CAD build for the part. Positions are in the model's coordinates, mm. A direction names the side the tool comes from. Give positions to 0.01 mm unless a question says otherwise; leave off trailing zeros. Loops run counter-clockwise (first coordinate to the right, second up) from the corner with the lowest first, then second, coordinate; pieces in that order, holes last. Notation, with made-up numbers: (17.25, 71.5) -> (55.25, 71.5) arc R26 cw to (55.25, 107.5) -> close; hole circle Ø2 at (-27, 24.5). An arc over 180 degrees is marked (long way). Use one line per item in the form item = value.
```python
from build123d import *

# Parameters (mm, degrees)
SKETCH1_R           = 77.4600051
BOSS_EXTRUDE1_DEPTH = 3.175
SKETCH24_R          = 22.1615
SKETCH24_R_2        = 2.0193
CUT_EXTRUDE14_DEPTH = 110.590991442


with BuildPart() as part:
    # Sketch1 → Boss-Extrude1 (new body)
    with BuildSketch(Plane(origin=(0, 0, 0), x_dir=(1, 0, 0), z_dir=(0, 1, 0))):
        with Locations(Location((0, 0, 0), (0, 0, 270))):
            Circle(SKETCH1_R)
    extrude(amount=BOSS_EXTRUDE1_DEPTH)

    # Sketch24 → Cut-Extrude14 (cut, through all)
    with BuildSketch(Plane(origin=(0, 3.175, 0), x_dir=(1, 0, 0), z_dir=(0, 1, 0))):
        with Locations(Location((0, 0, 0), (0, 0, 270))):
            Circle(SKETCH24_R)
        with Locations(Location((-25.4, 25.4, 0), (0, 0, 270))):
            Circle(SKETCH24_R_2)
        with Locations(Location((0, 33.02, 0), (0, 0, 270))):
            Circle(SKETCH24_R_2)
        with Locations(Location((33.02, 0, 0), (0, 0, 270))):
            Circle(SKETCH24_R_2)
        with Locations(Location((0, -33.02, 0), (0, 0, 270))):
            Circle(SKETCH24_R_2)
        with Locations(Location((-33.02, 0, 0), (0, 0, 270))):
            Circle(SKETCH24_R_2)
        with BuildLine():
            Line((-32.276051224, 28.683948776), (-41.256307345, 37.664204897))
            ThreePointArc((-41.256307345, 37.664204897), (-41.256307345, 41.256307345), (-37.664204897, 41.256307345))
            Line((-37.664204897, 41.256307345), (-28.683948776, 32.276051224))
            ThreePointArc((-28.683948776, 32.276051224), (-28.683948776, 28.683948776), (-32.276051224, 28.683948776))
        make_face()
        with BuildLine():
            Line((-27.903416949, -9.657564215), (-23.915755925, -17.31778977))
            ThreePointArc((-23.915755925, -17.31778977), (-26.616171022, -25.882412255), (-35.180793507, -23.181997158))
            Line((-35.180793507, -23.181997158), (-39.16845453, -15.521771603))
            ThreePointArc((-39.16845453, -15.521771603), (-36.468039434, -6.957149118), (-27.903416949, -9.657564215))
        make_face()
    extrude(amount=-CUT_EXTRUDE14_DEPTH, mode=Mode.SUBTRACT)


solid = part.part
```
1. Cut at A-A, the plane z = 0. Write the cut outline in (x, y) (1 decimal).
Result sheet:
outline = (-77.5, 0) -> (-35, 0) -> (-35, 3.2) -> (-77.5, 3.2) -> close; (-31, 0) -> (-22.2, 0) -> (-22.2, 3.2) -> (-31, 3.2) -> close; (22.2, 0) -> (31, 0) -> (31, 3.2) -> (22.2, 3.2) -> close; (35, 0) -> (77.5, 0) -> (77.5, 3.2) -> (35, 3.2) -> close
2. Cut at C-C, the plane y = 1.1. State how many separate pieces and enclosed holes the cut face has, then the cut area to 3 significant figures.
Result sheet:
separate_pieces = 1
enclosed_holes = 8
area = 16,900 mm^2
3. Cut at D-D, the plane x = 19.5. Write the cut outline in (y, z) (3 decimals), then the cut area to 3 significant figures.
Result sheet:
outline = (0, -74.965) -> (3.175, -74.965) -> (3.175, -10.53) -> (0, -10.53) -> close; (0, 10.53) -> (3.175, 10.53) -> (3.175, 74.965) -> (0, 74.965) -> close
area = 409 mm^2
4. Mould opens along X. For faces 1 (the flat face through (-16, 0, 16)), 2 (the cylindrical face through (-35, 1.6, -0.4)), 3 (the cylindrical face through (23.27, 1.57, 73.88)) say: pulls with the +X half, pulls with the -X half, needs draft (parallel to the pull), parting line crosses it, or undercut.
Result sheet:
face_1 = needs draft
face_2 = undercut
face_3 = parting line crosses it
5. Tool access for faces 4 (the flat face through (-16, 3.175, 16)), 5 (the flat face through (-36.7, 1.61, -33.11)): list every direction of +Z, -Z, +X, -X, +Y, -Y with a clear straight run to the whole face (end or side of a thin tool).
Result sheet:
face_4 = +Z, -Z, +X, -X, +Y
face_5 = +Y, -Y
6. Drop flat-ended pins along their axis: P1, Ø2.5, axis at x = -25.4, z = -25.4, coming from the +Y side; P2, Ø1, axis at x = -21.5, z = 18.5, coming from the -Y side. Give the stop position or say it passes through.
Result sheet:
P1 = through
P2 = 0
7. Drill centre lines: line 1 (X direction, y = 2.2, z = 0); line 2 (Z direction, x = -31.5, y = 0.3); line 3 (Z direction, x = -34.5, y = 2.6). Where is each one in solid material? Low to high.
Result sheet:
line_1 = -77.46 to -35.04, -31 to -22.16, 22.16 to 31, 35.04 to 77.46
line_2 = -70.77 to -35.09, -28.15 to -1.33, 1.33 to 6.57, 26.29 to 70.77
line_3 = -69.35 to -38.09, -30.91 to -1.37, 1.37 to 6.31, 24.23 to 69.35
8. Cut at B-B, the plane x = 0. Write the cut outline in (y, z) (1 decimal).
Result sheet:
outline = (0, -77.5) -> (3.2, -77.5) -> (3.2, -35) -> (0, -35) -> close; (0, -31) -> (3.2, -31) -> (3.2, -22.2) -> (0, -22.2) -> close; (0, 22.2) -> (3.2, 22.2) -> (3.2, 31) -> (0, 31) -> close; (0, 35) -> (3.2, 35) -> (3.2, 77.5) -> (0, 77.5) -> close
